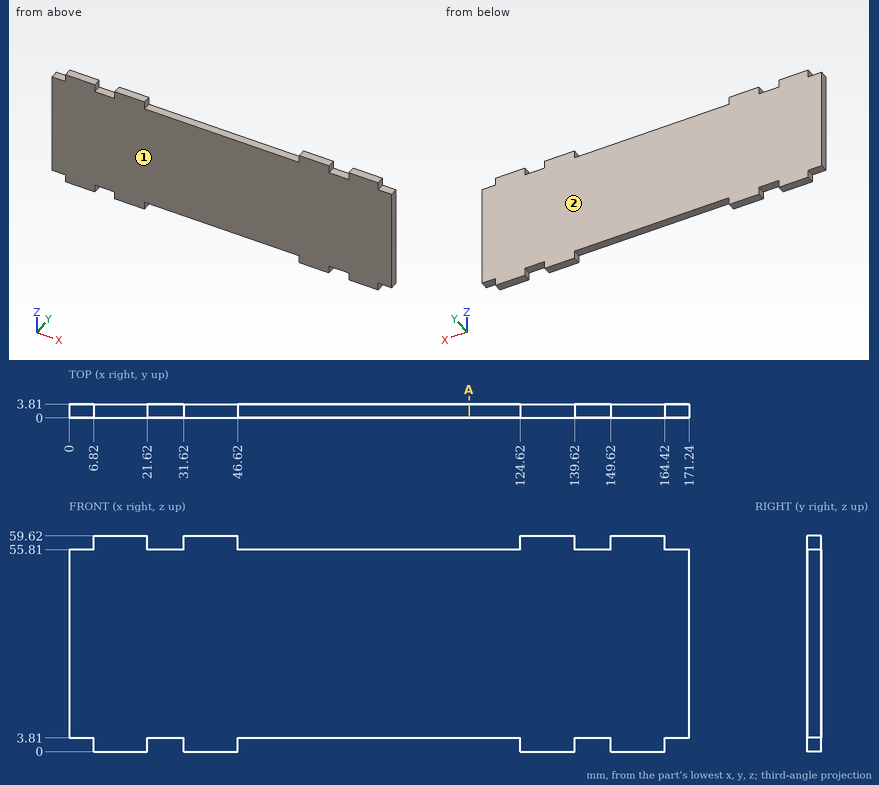
Check sheet for the drawn part. Datum: minimum x, y, z corner. Units: mm. Give positions to 0.01 mm unless a question says otherwise; leave off trailing zeros. Loops run counter-clockwise (first coordinate to the right, second up) from the corner with the lowest first, then second, coordinate; pieces in that order, holes last. Notation, with made-up numbers: M 5.25,-3 L 18.25,-3 A10 ccw 18.25,7 Z; hole C -22.5,17 d3. An arc over 180 degrees is marked long. Return JSON: item names as keys, results as strings.
1) Gauge pin test, flat ends, axial feed: P1, Ø1.1, axis at x = 3.5, y = 2.5, coming from the -Z side; P2, Ø1.9, axis at y = 2, z = 2, coming from the +X side; P3, Ø1.1, axis at x = 29, y = 2.5, coming from the +Z side. Record the tip position at first contact, or that the pin passes through.
Findings:
{"P1": "stops at z = 3.81", "P2": "stops at x = 164.42", "P3": "stops at z = 55.81"}
2) Mould release check, pull along Y, two halves, no side actions. Record for the marked faces 1 and 2: released by +Y, released by -Y, zero draft, split by the parting line, or undercut.
Findings:
{"face 1": "released by -Y", "face 2": "released by +Y"}
3) Section check A-A, the plane x = 110.5. Enter the section's corners in (y, z), and give its area (3 significant figures).
Findings:
{"outline": "M 0,3.81 L 3.81,3.81 L 3.81,55.81 L 0,55.81 Z", "area": "198 mm2"}
4) Material ranges on L1, parallel to X at y = 3.5, z = 57; L2, parallel to Z at x = 60.5, y = 0.65, recorded low to high. Write a range as [from, to].
Findings:
{"L1": "x = [6.82, 21.62], [31.62, 46.62], [124.62, 139.62], [149.62, 164.42]", "L2": "z = [3.81, 55.81]"}
